Part model, mm, in its own coordinate system. A direction names the side the tool comes from. Round coordinates to 2 decimals unless told otherwise and drop trailing zeros. Loops run counter-clockwise (first coordinate to the right, second up) from the corner with the lowest first, then second, coordinate; pieces in that order, holes last. Notation, with made-up numbers: (11, 84.5) - (41, 84.5) arc R15 ccw to (41, 99.5) - close; hole circle Ø10 at (29, 74). An arc over 180 degrees is marked (long way). Put each result on its own line as item: value.
from build123d import *

# Parameters (mm, degrees)
SKETCH1_W           = 104
SKETCH1_H           = 70
SKETCH1_W_2         = 100.5
SKETCH1_H_2         = 64.5
BOSS_EXTRUDE1_DEPTH = 21
CHAMFER2_SIZE       = 3.5
CHAMFER3_SIZE       = 5
SKETCH3_W           = 104
SKETCH3_H           = 70
BOSS_EXTRUDE2_DEPTH = 2
CHAMFER4_SIZE       = 5
SKETCH4_W           = 22
SKETCH4_H           = 31
CUT_EXTRUDE1_DEPTH  = 2
FILLET1_R           = 5


with BuildPart() as part:
    # Sketch1 → Boss-Extrude1 (new body)
    with BuildSketch(Plane(origin=(0, 0, 0), x_dir=(1, 0, 0), z_dir=(0, 1, 0))):
        Rectangle(SKETCH1_W, SKETCH1_H)
        Rectangle(SKETCH1_W_2, SKETCH1_H_2, mode=Mode.SUBTRACT)
    extrude(amount=BOSS_EXTRUDE1_DEPTH)

    # Chamfer2
    chamfer2_edges = [part.edges().sort_by_distance(p)[0] for p in [
        (50.25, 10.5, 32.25),
        (50.25, 10.5, -32.25),
        (-50.25, 10.5, -32.25),
        (-50.25, 10.5, 32.25),
    ]]
    chamfer(chamfer2_edges, length=CHAMFER2_SIZE)

    # Chamfer3
    chamfer3_edges = [part.edges().sort_by_distance(p)[0] for p in [
        (52, 10.5, 35),
        (-52, 10.5, 35),
        (-52, 10.5, -35),
        (52, 10.5, -35),
    ]]
    chamfer(chamfer3_edges, length=CHAMFER3_SIZE)

    # Sketch3 → Boss-Extrude2 (add)
    with BuildSketch(Plane(origin=(0, 21, 0), x_dir=(1, 0, 0), z_dir=(0, 1, 0))):
        Rectangle(SKETCH3_W, SKETCH3_H)
    extrude(amount=BOSS_EXTRUDE2_DEPTH)

    # Chamfer4
    chamfer4_edges = [part.edges().sort_by_distance(p)[0] for p in [
        (-52, 22, 35),
        (52, 22, 35),
        (52, 22, -35),
        (-52, 22, -35),
    ]]
    chamfer(chamfer4_edges, length=CHAMFER4_SIZE - 0.0001)  # a hair under: the kernel refuses the full size

    # Sketch4 → Cut-Extrude1 (cut)
    with BuildSketch(Plane.XZ.offset(-21)):
        with Locations((0, 0.5)):
            Rectangle(SKETCH4_W, SKETCH4_H)
        with Locations((33, 0.5)):
            Rectangle(SKETCH4_W, SKETCH4_H)
        with Locations((-33, 0.5)):
            Rectangle(SKETCH4_W, SKETCH4_H)
    extrude(amount=-CUT_EXTRUDE1_DEPTH, mode=Mode.SUBTRACT)

    # Fillet1
    fillet1_edges = [part.edges().sort_by_distance(p)[0] for p in [
        (-11, 22, -15),
        (-11, 22, 16),
        (11, 22, 16),
        (11, 22, -15),
        (22, 22, -15),
        (22, 22, 16),
        (44, 22, 16),
        (44, 22, -15),
        (-22, 22, 16),
        (-22, 22, -15),
        (-44, 22, -15),
        (-44, 22, 16),
    ]]
    fillet(fillet1_edges, radius=FILLET1_R)


solid = part.part
1. Band-saw the part on A-A (x = -2). List the corners of the cut face in (y, z), plus the area to 4 significant figures.
A:
outline: (0, -35) - (23, -35) - (23, -15) - (21, -15) - (21, -32.25) - (0, -32.25) - close; (0, 32.25) - (21, 32.25) - (21, 16) - (23, 16) - (23, 35) - (0, 35) - close
area: 193.5 mm²
2. Band-saw the part on B-B (z = -11.5). List the corners of the cut face in (x, y), plus the area to 3 significant figures.
A:
outline: (-52, 0) - (-50.25, 0) - (-50.25, 21) - (-43.77, 21) - (-43.77, 23) - (-52, 23) - close; (-22.23, 21) - (-10.77, 21) - (-10.77, 23) - (-22.23, 23) - close; (10.77, 21) - (22.23, 21) - (22.23, 23) - (10.77, 23) - close; (43.77, 21) - (50.25, 21) - (50.25, 0) - (52, 0) - (52, 23) - (43.77, 23) - close
area: 152 mm²
3. Tool access for faces 1 (the flat face through (50, 10, -32)), 2 (the flat face through (49, 10, 30)), 3 (the cylindrical face through (-43, 22, 14)): list every direction of +Z, -Z, +X, -X, +Y, -Y with a clear straight run to the whole face (end or side of a thin tool).
A:
face 1: -Z, +X, +Y, -Y
face 2: -Y
face 3: +Y, -Y
4. Probe line 1 along X through (y, z) = (8, -20); line 2 along Z through (x, y) = (43, 12.5); line 3 along Y through (x, z) = (21, 15.5). List the from-to ranges inside material, lowest first. Write a range as [from, to].
A:
line 1: x = [-52, -50.25], [50.25, 52]
line 2: z = [-35, -32.25], [32.25, 35]
line 3: y = [21, 23]
5. Band-saw the part on D-D (x = 16). List the corners of the cut face in (y, z), plus the area to 4 significant figures.
A:
outline: (0, -35) - (23, -35) - (23, 35) - (0, 35) - (0, 32.25) - (21, 32.25) - (21, -32.25) - (0, -32.25) - close
area: 255.5 mm²
6. Pin check, flat tip, straight feed: P1, Ø5, axis at x = 23.5, z = 8, coming from the -Y side. Stop position of the tip, or through.
A:
P1: stops at y = 21
7. Two-plate mould, pull along Z, no slides. Class faces 4 (the flat face through (-49, 22, -33)), 5 (the flat face through (-49, 22, 33)), 6 (the cylindrical face through (10, 22, -13)), 7 (the flat face through (-52, 11, 0)): pulls with the +Z half, pulls with the -Z half, needs draft (parallel to the pull), parting line crosses it, or undercut.
A:
face 4: pulls with the -Z half
face 5: pulls with the +Z half
face 6: undercut
face 7: needs draft
8. Band-saw the part on C-C (y = 8). List the corners of the cut face in (x, z).
A:
outline: (-52, -30) - (-47, -35) - (47, -35) - (52, -30) - (52, 30) - (47, 35) - (-47, 35) - (-52, 30) - close; hole (-50.25, -28.75) - (-46.75, -32.25) - (46.75, -32.25) - (50.25, -28.75) - (50.25, 28.75) - (46.75, 32.25) - (-46.75, 32.25) - (-50.25, 28.75) - close
